Geometry check sheet. Reference: the model listing, model coordinates, mm. A direction names the side the tool comes from. Round coordinates to 2 decimals unless told otherwise and drop trailing zeros. Order: outer loops, then holes, each group sorted by start corner. A loop starts at its lowest first (then second) coordinate and runs counter-clockwise, first axis right, second up. Notation, with made-up numbers: (39.25, -6) -> (75.25, -6) arc R22 ccw to (75.25, 5) -> close; hole circle Ø2 at (67, -30). An arc over 180 degrees is marked (long way). Answer as a JSON object with one key per item and string values. Group by question number.
from build123d import *

# Parameters (mm, degrees)
SALIENTE_EXTRUIR1_DEPTH = 3.9
CORTAR_EXTRUIR1_DEPTH   = 2.1


with BuildPart() as part:
    # Croquis1 → Saliente-Extruir1 (new body)
    with BuildSketch(Plane.XY):
        with BuildLine():
            Line((0, 0), (-12, 0))
            Line((-12, 0), (-12, 9.5341439))
            ThreePointArc((-12, 9.5341439), (-15.903544777, 12.873087069), (-18.1346611, 17.5))
            Line((-18.1346611, 17.5), (-26.5, 17.5))
            Line((-26.5, 17.5), (-26.5, 23.5))
            Line((-26.5, 23.5), (-18.1346611, 23.5))
            ThreePointArc((-18.1346611, 23.5), (-14.838834765, 29.338834765), (-9, 32.6346611))
            Line((-9, 32.6346611), (-9, 41))
            Line((-9, 41), (-3, 41))
            Line((-3, 41), (-3, 32.6346611))
            ThreePointArc((-3, 32.6346611), (2.838834765, 29.338834765), (6.1346611, 23.5))
            Line((6.1346611, 23.5), (14.5, 23.5))
            Line((14.5, 23.5), (14.5, 17.5))
            Line((14.5, 17.5), (6.1346611, 17.5))
            ThreePointArc((6.1346611, 17.5), (3.903544777, 12.873087069), (0, 9.5341439))
            Line((0, 9.5341439), (0, 0))
        make_face()
        with BuildLine():
            Line((-9, 23.5), (-9, 27.373863542))
            ThreePointArc((-9, 27.373863542), (-11.303300859, 25.803300859), (-12.873863542, 23.5))
            Line((-12.873863542, 23.5), (-9, 23.5))
        make_face(mode=Mode.SUBTRACT)
        with BuildLine():
            Line((-3, 23.5), (-3, 27.373863542))
            ThreePointArc((-3, 27.373863542), (-0.696699141, 25.803300859), (0.873863542, 23.5))
            Line((0.873863542, 23.5), (-3, 23.5))
        make_face(mode=Mode.SUBTRACT)
        with BuildLine():
            Line((-9, 17.5), (-9, 13.626136458))
            ThreePointArc((-9, 13.626136458), (-11.303300859, 15.196699141), (-12.873863542, 17.5))
            Line((-12.873863542, 17.5), (-9, 17.5))
        make_face(mode=Mode.SUBTRACT)
        with BuildLine():
            Line((-3, 17.5), (-3, 13.626136458))
            ThreePointArc((-3, 13.626136458), (-0.696699141, 15.196699141), (0.873863542, 17.5))
            Line((0.873863542, 17.5), (-3, 17.5))
        make_face(mode=Mode.SUBTRACT)
    extrude(amount=SALIENTE_EXTRUIR1_DEPTH)

    # Croquis2 → Cortar-Extruir1 (cut)
    with BuildSketch(Plane.XY.offset(3.9)):
        with BuildLine():
            Line((-10.6, 0), (-1.4, 0))
            Line((-1.4, 0), (-1.4, 6.5))
            ThreePointArc((-1.4, 6.5), (-2.021320344, 8), (-1.4, 9.5))
            Line((-1.4, 9.5), (-1.4, 12))
            Line((-1.4, 12), (-10.6, 12))
            Line((-10.6, 12), (-10.6, 9.5))
            ThreePointArc((-10.6, 9.5), (-9.978679656, 8), (-10.6, 6.5))
            Line((-10.6, 6.5), (-10.6, 0))
        make_face()
    extrude(amount=-CORTAR_EXTRUIR1_DEPTH, mode=Mode.SUBTRACT)


solid = part.part
Item 1: Sectioned sample at A-A, the plane z = 0.65. Enter the section's corners in (x, y).
Item 2: Sectioned sample at C-C, the plane y = 8. Enter the section's corners in (x, z), then the cut area to 3 significant figures.
Item 3: Sectioned sample at D-D, the plane x = -20. Enter the section's corners in (y, z), then the cut area to 3 significant figures.
Item 4: Thickness scan on L1, parallel to X at y = 5.5, z = 2.9; L2, parallel to Y at x = -24, z = 1.55; L3, parallel to Y at x = -10.5, z = 2.85. Record the ranges inside material, lowest first.
Item 5: Depth check by flat-ended pin: pin 1 Ø4.5 at (x, y) = (-7.5, 4.5) entering from +Z; pin 2 Ø1.9 at (y, z) = (25.5, 1.5) entering from +X; pin 3 Ø1.7 at (y, z) = (4, 3) entering from +X; pin 4 Ø3 at (x, y) = (-11, 35.5) entering from +Z. Enter the tip coordinate at first touch or a pass-through.
Item 6: Sectioned sample at B-B, the plane y = 24. Enter the section's corners in (x, z).
Item 7: Set-up check for faces 1 (the flat face through (-11, 23.5, 2)), 2 (the flat face through (-1.4, 11, 3)): record each of +Z, -Z, +X, -X, +Y, -Y from which the full face is reachable in a straight line by a thin tool's end or side.
Item 8: Mould release check, pull along Y, two halves, no side actions. Record for faces 3 (the cylindrical face through (4, 13, 2)), 4 (the flat face through (-9, 37, 2)), 5 (the flat face through (-1, 23.5, 2)): pulls with the +Y half, pulls with the -Y half, needs draft (parallel to the pull), parting line crosses it, or undercut.
Result:
{
 "1": {"outline": "(-26.5, 17.5) -> (-18.13, 17.5) arc R12.5 ccw to (-12, 9.53) -> (-12, 0) -> (0, 0) -> (0, 9.53) arc R12.5 ccw to (6.13, 17.5) -> (14.5, 17.5) -> (14.5, 23.5) -> (6.13, 23.5) arc R12.5 ccw to (-3, 32.63) -> (-3, 41) -> (-9, 41) -> (-9, 32.63) arc R12.5 ccw to (-18.13, 23.5) -> (-26.5, 23.5) -> close; hole (-12.87, 17.5) arc R7.5 ccw to (-9, 13.63) -> (-9, 17.5) -> close; hole (-12.87, 23.5) -> (-9, 23.5) -> (-9, 27.37) arc R7.5 ccw to start; hole (-3, 13.63) arc R7.5 ccw to (0.87, 17.5) -> (-3, 17.5) -> close; hole (-3, 23.5) -> (0.87, 23.5) arc R7.5 ccw to (-3, 27.37) -> close"},
 "2": {"outline": "(-12, 0) -> (0, 0) -> (0, 3.9) -> (-2.02, 3.9) -> (-2.02, 1.8) -> (-9.98, 1.8) -> (-9.98, 3.9) -> (-12, 3.9) -> close", "area": "30.1 mm2"},
 "3": {"outline": "(17.5, 0) -> (23.5, 0) -> (23.5, 3.9) -> (17.5, 3.9) -> close", "area": "23.4 mm2"},
 "4": {"L1": "x = -12 to -10.6, -1.4 to 0", "L2": "y = 17.5 to 23.5", "L3": "y = 6.61 to 9.39, 12 to 14.5, 17.5 to 23.5, 26.5 to 32.16"},
 "5": {"pin 1": "stops at z = 1.8", "pin 2": "stops at x = 5.83", "pin 3": "stops at x = 0", "pin 4": "passes through"},
 "6": {"outline": "(-18, 0) -> (-12.63, 0) -> (-12.63, 3.9) -> (-18, 3.9) -> close; (-9, 0) -> (-3, 0) -> (-3, 3.9) -> (-9, 3.9) -> close; (0.63, 0) -> (6, 0) -> (6, 3.9) -> (0.63, 3.9) -> close"},
 "7": {"face 1": "+Z, -Z", "face 2": "+Z"},
 "8": {"face 3": "pulls with the -Y half", "face 4": "needs draft", "face 5": "undercut"}
}
